Source: CAD feature listing. Evaluate the final solid. Frame: model axes, mm. A direction names the side the tool comes from. Give positions to 0.01 mm unless a question says otherwise; leave off trailing zeros. Write each loop counter-clockwise with the first axis right and the second up, starting at its lowest first coordinate (ties: lowest second). Pieces come first, ordered by that corner, then holes. Notation, with made-up numbers: M -27,-1.75 L 12,-1.75 A5 cw 12,5.25 Z; hole C -23,69 d6. An arc over 180 degrees is marked long. Use CSV: the item, a comma, the result in double quotes. Start each with the question number.
Autodesk Inventor part; units mm, degrees
ref_plane "YZ Plane" through (0, 0, 0) normal (1, 0, 0) x (0, 1, 0)
ref_plane "XZ Plane" through (0, 0, 0) normal (0, 1, 0) x (-1, 0, 0)
ref_plane "XY Plane" through (0, 0, 0) normal (0, 0, 1) x (1, 0, 0)
sketch "Sketch1" plane through (0, 0, 0) normal (0, 1, 0) x (-1, 0, 0)
  circle A0 centre (0, 0) radius 4.35
  dimension "d0" = 8.7
extrude "Extrusion1" add sketch "Sketch1" along normal blind 6
sketch "Sketch2" plane through (0, 6, 0) normal (0, 1, 0) x (1, 0, 0)
  circle A0 centre (0, 0) radius 3
  dimension "d3" = 6
extrude "Extrusion2" add sketch "Sketch2" along normal blind 5
fillet "Fillet1" radius 2 1 edges at (-3, 6, 0)
sketch "Sketch3" plane through (0, 0, 0) normal (0, -1, 0) x (1, 0, 0)
  line L0 (-10, -10) -> (10, -10)
  line L1 (10, -10) -> (10, 10)
  line L2 (10, 10) -> (-10, 10)
  line L3 (-10, 10) -> (-10, -10)
  line L4 (-10, -10) -> (10, 10) construction
  line L5 (10, -10) -> (-10, 10) construction
  point P0 (0, 0)
  dimension "d7" = 20
  dimension "d8" = 20
extrude "Extrusion3" add sketch "Sketch3" along normal blind 4
sketch "Sketch4" plane through (0, 0, 0) normal (0, 1, 0) x (1, 0, 0)
  circle A0 centre (0, 0) radius 3
  circle A1 centre (0, 0) radius 7.5
  circle A2 centre (-7.5, 0) radius 1
  circle A3 centre (0, -7.5) radius 1
  circle A4 centre (7.5, 0) radius 1
  circle A5 centre (0, 7.5) radius 1
  dimension "d11" = 15
  dimension "d12" = 2
  dimension "d15" = 360
hole "Hole1" at (-7.5, 0, 0) at (0, 0, 7.5) at (7.5, 0, 0) at (0, 0, -7.5) direction (0, -1, 0) diameter 2 end through all
fillet "Fillet2" radius 2 2 edges at (0, 6, -4.35) (0, 6, 4.35)
equation "\"d22\" = Thickness"
equation "\"BendRadius\" = Thickness"
equation "\"BendReliefWidth\" = Thickness"
equation "\"BendReliefDepth\" = 0.5 * Thickness"
equation "\"CornerReliefSize\" = 4 * Thickness"
equation "\"MinimumRemnant\" = 2 * Thickness"
equation "\"TransitionRadius\" = BendRadius"
equation "\"JacobiRadiusSize\" = BendRadius"
equation "\"GapSize\" = Thickness"
properties part number "placeHolder"
Item 1: Section D-D (x = -5). Return the cut outline in (y, z).
Item 2: Contact query for flat-ended pins moving along their axis: pin 1 Ø1.8 at (x, z) = (-7.5, 0) entering from +Y; pin 2 Ø1 at (x, y) = (-1.5, 4) entering from -Z; pin 3 Ø6 at (y, z) = (4.5, -4.5) entering from +X; pin 4 Ø1.5 at (x, y) = (-1.5, 4) entering from +Z. Output: stop coordinate, or through.
Item 3: Section A-A (z = 7.5). Return the cut outline in (x, y).
Item 4: Set-up query: faces 1 (the cylindrical face through (-3, 9, 0)), 2 (the cylindrical face through (6.51, -2.03, -0.13)). Return all of +Z, -Z, +X, -X, +Y, -Y with unobstructed straight access to the full face (end or side cutting, diameter ignored); none if empty.
Item 5: Section C-C (x = 0.5). State how many separate pieces and enclosed holes the cut face has, plus the area to 3 significant figures.
Item 6: Pull-direction query (Z, two-part tool) for faces 3 (the flat face through (0, -4, 0)), 4 (the cylindrical face through (0.943, 2.413, 4.247)), 5 (the cylindrical face through (0.6, -2, -8.3)); classes: released by +Z, released by -Z, zero draft, split by the parting line, or undercut.
Item 7: Section B-B (y = 8.75). Return the cut outline in (x, z).
Item 8: Material intervals for probe 1 along X at (y, z) = (-1.4, 0); probe 2 along X at (y, z) = (-2.3, 7.5), sorted ascending.
Output values:
1,outline,"M -4,-10 L 0,-10 L 0,10 L -4,10 Z"
2,pin 1,"passes through"
2,pin 2,"stops at z = -4.23"
2,pin 3,"stops at x = 4.08"
2,pin 4,"stops at z = 4.28"
3,outline,"M -10,-4 L -1,-4 L -1,0 L -10,0 Z; M 1,-4 L 10,-4 L 10,0 L 1,0 Z"
4,face 1,"+Y"
4,face 2,"+Y, -Y"
5,separate pieces,"3"
5,enclosed holes,"0"
5,area,"149 mm2"
6,face 3,"zero draft"
6,face 4,"split by the parting line"
6,face 5,"undercut"
7,outline,"C 0,0 d6"
8,probe 1,"x = -10 to -8.5, -6.5 to 6.5, 8.5 to 10"
8,probe 2,"x = -10 to -1, 1 to 10"
